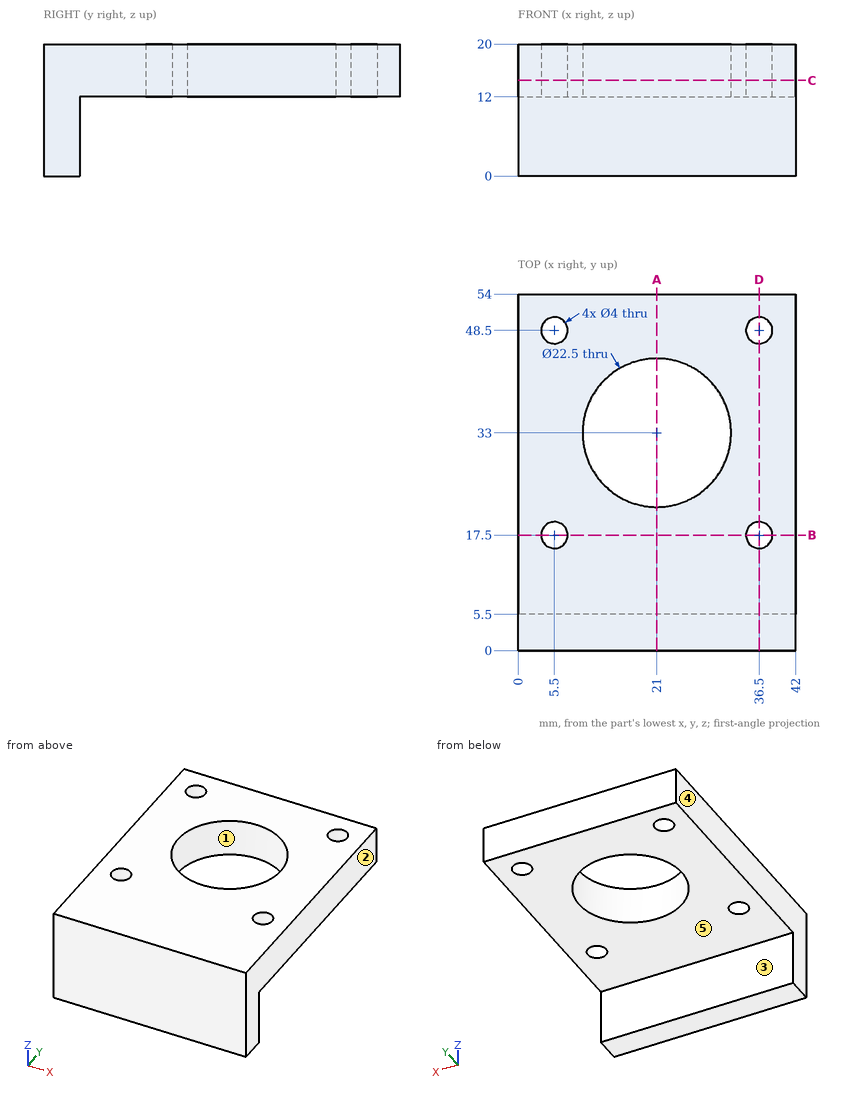
The figure shows three views and two pictorial views of one solid part (mm, origin at its lowest corner). Answer the questions. A direction names the side the tool comes from. Give positions to 0.01 mm unless a question says otherwise; leave off trailing zeros. Write each loop counter-clockwise with the first axis right and the second up, starting at its lowest first coordinate (ties: lowest second). Pieces come first, ordered by that corner, then holes. Notation, with made-up numbers: (80, 59.25) - (100, 59.25) arc R26 cw to (100, 78.25) - close; hole circle Ø6 at (10.25, -22). An arc over 180 degrees is marked (long way). Use CSV: the item, a comma, the result in double quotes. Start each with the question number.
Item 1: The part is cut by section A-A, the plane x = 21. Give the vertices of the cut face in (y, z), and give its area (3 significant figures).
Item 2: The part is cut by section D-D, the plane x = 36.5. Give the vertices of the cut face in (y, z), and give its area (3 significant figures).
Item 3: The part is cut by section B-B, the plane y = 17.5. Give the vertices of the cut face in (x, z), and give its area (3 significant figures).
Item 4: Flat-ended cylindrical pins translate along their axes: P1, Ø10, axis at y = 29.5, z = 12.5, coming from the -X side; P2, Ø3.5, axis at x = 29, z = 8.5, coming from the +Y side; P3, Ø6.5, axis at x = 5.5, y = 48.5, coming from the -Z side. Find the tip coordinate at first contact, or state that the pin passes through.
Item 5: For the marked faces 4 and 5, determine the directions among +Z, -Z, +X, -X, +Y, -Y from which every point of the face is accessible in a straight line to the end or side of a thin tool.
Item 6: The part is cut by section C-C, the plane z = 14.5. Give the vertices of the cut face in (x, y), and give its area (3 significant figures).
Item 7: The mould has two halves that part along X. Classify the marked faces 1, 2 and 3: pulls with the +X half, pulls with the -X half, needs draft (parallel to the pull), parting line crosses it, or undercut.
Item 8: Consider line 1 (Y direction, x = 5.5, z = 15.75); line 2 (Y direction, x = 38, z = 14.5); line 3 (X direction, y = 50, z = 19). Determine where each line is inside the solid, lowest interval first.
Taken from the geometry:
1,outline,"(0, 0) - (5.5, 0) - (5.5, 12) - (21.75, 12) - (21.75, 20) - (0, 20) - close; (44.25, 12) - (54, 12) - (54, 20) - (44.25, 20) - close"
1,area,"318 mm2"
2,outline,"(0, 0) - (5.5, 0) - (5.5, 12) - (15.5, 12) - (15.5, 20) - (0, 20) - close; (19.5, 12) - (46.5, 12) - (46.5, 20) - (19.5, 20) - close; (50.5, 12) - (54, 12) - (54, 20) - (50.5, 20) - close"
2,area,"434 mm2"
3,outline,"(0, 12) - (3.5, 12) - (3.5, 20) - (0, 20) - close; (7.5, 12) - (34.5, 12) - (34.5, 20) - (7.5, 20) - close; (38.5, 12) - (42, 12) - (42, 20) - (38.5, 20) - close"
3,area,"272 mm2"
4,P1,"x = 0"
4,P2,"y = 5.5"
4,P3,"z = 12"
5,face 4,"+Z, -Z, -X, +Y, -Y"
5,face 5,"-Z, +X, -X, +Y"
6,outline,"(0, 0) - (42, 0) - (42, 54) - (0, 54) - close; hole circle Ø4 at (5.5, 17.5); hole circle Ø4 at (5.5, 48.5); hole circle Ø22.5 at (21, 33); hole circle Ø4 at (36.5, 17.5); hole circle Ø4 at (36.5, 48.5)"
6,area,"1,820 mm2"
7,face 1,"undercut"
7,face 2,"pulls with the +X half"
7,face 3,"needs draft"
8,line 1,"0 to 15.5, 19.5 to 46.5, 50.5 to 54"
8,line 2,"0 to 16.18, 18.82 to 47.18, 49.82 to 54"
8,line 3,"0 to 4.18, 6.82 to 35.18, 37.82 to 42"
